```python
from build123d import *

# Parameters (mm, degrees)
F0_W          = 130
F0_H          = 190
F2_DEPTH      = 120
F3_T          = -5
F5_DEPTH      = 95.001
F5_DEPTH_BACK = 95.001
F6_W          = 130
F6_H          = 30
F7_DEPTH      = 3
F8_W          = 30
F8_H          = 123
F9_DEPTH      = 3


# Not quite as in the source:
# - a pattern or mirror of a feature is missing from the dataset's text; its kind, count and spacing are read off the source's solid


with BuildPart() as f2:
    # F0 (on Top) → F2 (new body, through all)
    with BuildSketch(Plane.XY):
        Rectangle(F0_W, F0_H)
    extrude(amount=F2_DEPTH)

    # F3
    f3_openings = [f2.faces().sort_by_distance(p)[0] for p in [
        (0, 0, 120),
    ]]
    offset(amount=F3_T, openings=f3_openings)

    # F4 (on Front) → F5 (cut, two sides)
    with BuildSketch(Plane.XZ) as f5_sk:
        with BuildLine():
            Line((30, 100), (-30, 100))
            ThreePointArc((-30, 100), (-36, 94), (-30, 88))
            Line((-30, 88), (30, 88))
            ThreePointArc((30, 88), (36, 94), (30, 100))
        make_face()
    extrude(amount=-F5_DEPTH, mode=Mode.SUBTRACT)
    extrude(f5_sk.sketch, amount=F5_DEPTH_BACK, mode=Mode.SUBTRACT)

    # F6 (on face) → F7 (join)
    with BuildSketch(Plane(origin=(0, 0, 0), x_dir=(1, 0, 0), z_dir=(0, 0, -1))):
        with Locations((0, 60)):
            Rectangle(F6_W, F6_H)
        with Locations((0, -60)):
            Rectangle(F6_W, F6_H)
    extrude(amount=F7_DEPTH)

    # F8 (on face) → F9 (join)
    with BuildSketch(Plane.YZ.offset(65)):
        with Locations((-60, 58.5)):
            Rectangle(F8_W, F8_H)
        with Locations((60, 58.5)):
            Rectangle(F8_W, F8_H)
    f9 = extrude(amount=F9_DEPTH)

    # F9_copies: F9 across plane
    add(f9.mirror(Plane(origin=(0, 0, 0), x_dir=(0, 0, -1), z_dir=(-1, 0, 0))))


solid = f2.part
```
The model under review builds one solid part; all positions refer to its coordinate system, in mm. A direction names the side the tool comes from. Round coordinates to 2 decimals unless told otherwise and drop trailing zeros. Order: outer loops, then holes, each group sorted by start corner. A loop starts at its lowest first (then second) coordinate and runs counter-clockwise, first axis right, second up.
Item 1: Add section C-C, the plane y = -72. State the section outline as (x, z) points, and give its area (3 significant figures).
Working result:
outline: (-68, -3) - (68, -3) - (68, 120) - (60, 120) - (60, 5) - (-60, 5) - (-60, 120) - (-68, 120) - close
area: 2,930 mm2
Item 2: Draft analysis for pull direction Y (two halves, no side actions). For faces 4 (the flat face through (-1, 95, 59)), 5 (the cylindrical face through (-36, -92, 94)), 6 (the flat face through (-0.3, 45, -0.4)), state which applies: released by +Y, released by -Y, zero draft, split by the parting line, or undercut.
Working result:
face 4: released by +Y
face 5: zero draft
face 6: undercut
Item 3: Add section B-B, the plane z = 24.5. State the section outline as (x, y) points, and give its area (3 significant figures).
Working result:
outline: (-68, -75) - (-65, -75) - (-65, -95) - (65, -95) - (65, -75) - (68, -75) - (68, -45) - (65, -45) - (65, 45) - (68, 45) - (68, 75) - (65, 75) - (65, 95) - (-65, 95) - (-65, 75) - (-68, 75) - (-68, 45) - (-65, 45) - (-65, -45) - (-68, -45) - close; hole (-60, -90) - (60, -90) - (60, 90) - (-60, 90) - close
area: 3,460 mm2
Item 4: For pin 1 (16 mm diameter, centred on x = -16, y = -88, fed in from -Z); pin 2 (12 mm diameter, centred on x = 22, y = -2, fed in from +Z), all flat-tipped, find the tip position at first contact; note any pin that passes through.
Working result:
pin 1: stops at z = 0
pin 2: stops at z = 5
Item 5: Add section A-A, the plane x = 20. State the section outline as (y, z) points.
Working result:
outline: (-95, 0) - (-75, 0) - (-75, -3) - (-45, -3) - (-45, 0) - (45, 0) - (45, -3) - (75, -3) - (75, 0) - (95, 0) - (95, 88) - (90, 88) - (90, 5) - (-90, 5) - (-90, 88) - (-95, 88) - close; (-95, 100) - (-90, 100) - (-90, 120) - (-95, 120) - close; (90, 100) - (95, 100) - (95, 120) - (90, 120) - close
Item 6: To check wall thickness, follow probe 1 along Y at (x, z) = (56.5, 32); probe 2 along X at (y, z) = (24.5, 99); probe 3 along X at (y, z) = (45.5, 64). State the ranges of each line that lie inside material, in increasing order.
Working result:
probe 1: y = -95 to -90, 90 to 95
probe 2: x = -65 to -60, 60 to 65
probe 3: x = -68 to -60, 60 to 68
Item 7: Machinability: for faces 1 (the flat face through (-65, -1, 59)), 2 (the flat face through (60, -1, 62)), 3 (the cylindrical face through (36, -92, 94)), which of the approach directions +Z, -Z, +X, -X, +Y, -Y give a long, thin tool a straight path to every point of the face, cutting with its end or side? Answer none if there is none.
Working result:
face 1: +Z, -Z, -X
face 2: +Z
face 3: +Y, -Y
